Input: part model. Units: mm. Frame: model coordinates. Round coordinates to 2 decimals unless told otherwise and drop trailing zeros. Loops run counter-clockwise (first coordinate to the right, second up) from the corner with the lowest first, then second, coordinate; pieces in that order, holes last. Notation, with made-up numbers: M 58.5,78.25 L 76.5,78.25 A20 cw 76.5,94.25 Z; hole C 54.5,-22 d4. An arc over 180 degrees is marked long. Return JSON: item names as keys, results as strings. Group by question number.
1) Section B-B (x = -0.5). Output: boundary loops of the cut face in (y, z).
2) Material intervals for line 1 (X direction, y = -2.5, z = 0.1); line 2 (Y direction, x = -5, z = -0.1), sorted ascending. Write a range as from..to.
3) Section A-A (z = 0). Output: boundary loops of the cut face in (x, y).
4) Section D-D (x = 5.25). Output: boundary loops of the cut face in (y, z), plus the area to 3 significant figures.
from build123d import *

# Parameters (mm, degrees)
BOSS_EXTRUDE1_DEPTH = 0.254
CIRPATTERN2_COUNT   = 4


with BuildPart() as part:
    # Sketch3 → Boss-Extrude1 (new, symmetric)
    with BuildSketch(Plane.XY):
        with BuildLine():
            Line((4.2418, 0.762), (6.096, 0.762))
            Line((6.096, 0.762), (6.096, 4.572))
            ThreePointArc((6.096, 4.572), (5.649630735, 5.649630735), (4.572, 6.096))
            Line((4.572, 6.096), (-0.889, 6.096))
            Line((-0.889, 6.096), (-0.889, 4.2418))
            Line((-0.889, 4.2418), (3.8608, 4.2418))
            ThreePointArc((3.8608, 4.2418), (4.130207684, 4.130207684), (4.2418, 3.8608))
            Line((4.2418, 3.8608), (4.2418, 0.762))
        make_face()
    boss_extrude1 = extrude(amount=BOSS_EXTRUDE1_DEPTH, both=True)

    # CirPattern2: Boss-Extrude1 ×4 about axis
    cirpattern2_axis = Axis((0, 0, 0), (0, 0, 1))
    for i in range(1, CIRPATTERN2_COUNT):
        add(boss_extrude1.rotate(cirpattern2_axis, i * 360 / CIRPATTERN2_COUNT))


solid = part.part
Returned:
{
 "1": {"outline": "M -6.1,-0.25 L -4.24,-0.25 L -4.24,0.25 L -6.1,0.25 Z; M 4.24,-0.25 L 6.1,-0.25 L 6.1,0.25 L 4.24,0.25 Z"},
 "2": {"line 1": "x = -6.1..-4.24, 4.24..6.1", "line 2": "y = -6.03..6.03"},
 "3": {"outline": "M -6.1,-4.57 A1.52 ccw -4.57,-6.1 L 4.57,-6.1 A1.52 ccw 6.1,-4.57 L 6.1,4.57 A1.52 ccw 4.57,6.1 L -4.57,6.1 A1.52 ccw -6.1,4.57 Z; hole M -4.24,-3.86 A0.38 ccw -3.86,-4.24 L 3.86,-4.24 A0.38 ccw 4.24,-3.86 L 4.24,3.86 A0.38 ccw 3.86,4.24 L -3.86,4.24 A0.38 ccw -4.24,3.86 Z"},
 "4": {"outline": "M -5.94,-0.25 L 5.94,-0.25 L 5.94,0.25 L -5.94,0.25 Z", "area": "6.03 mm^2"}
}
